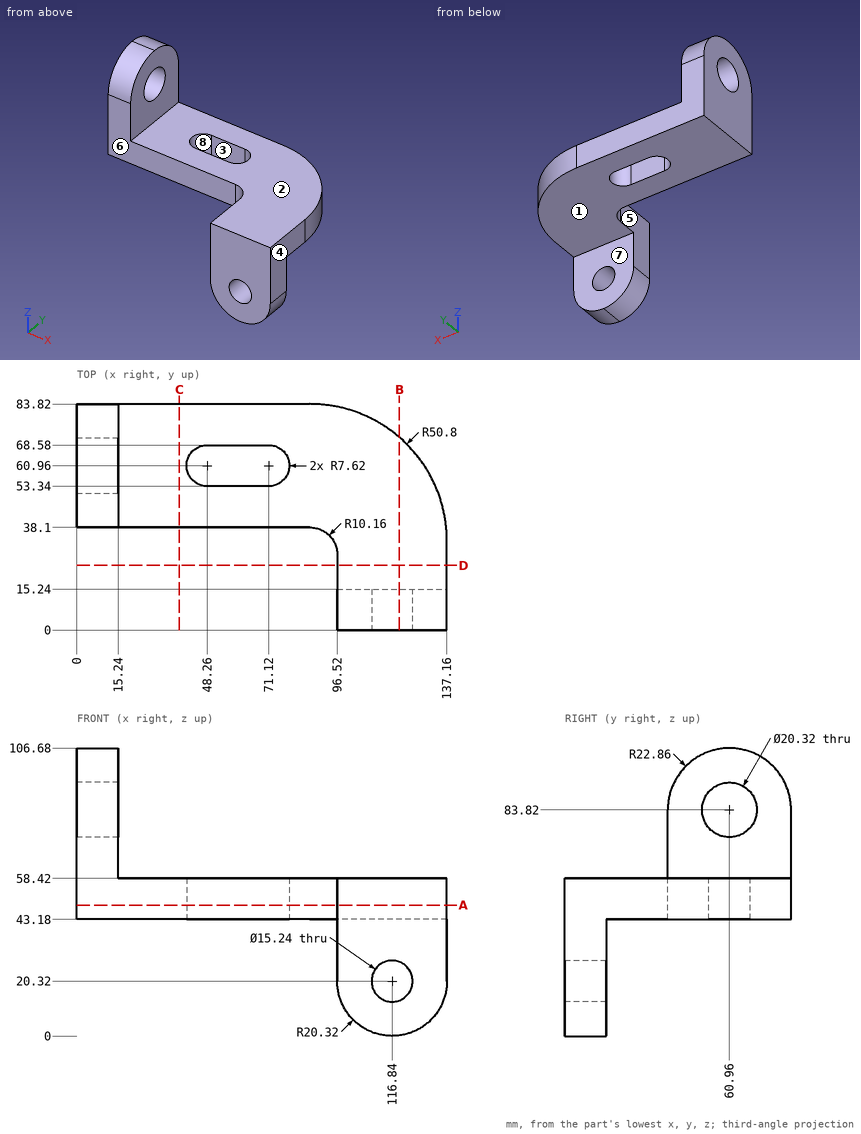
The figure shows three views and two pictorial views of one solid part (mm, origin at its lowest corner). Answer the questions. A direction names the side the tool comes from. Coordinates: 2 decimals unless noted, no trailing zeros. Order: outer loops, then holes, each group sorted by start corner. A loop starts at its lowest first (then second) coordinate and runs counter-clockwise, first axis right, second up.
Q1. A cutting plane is placed at D-D, the plane y = 24. Write down the section's boundary in (x, z), and give its area (3 significant figures).
Q2. Which of the six approach directions +Z, -Z, +X, -X, +Y, -Y give full straight-line access (tool end or side, diameter ignored) to the marked faces 1, 2, 3 and 4?
Q3. For a pull along Y with two mould halves and no side action, classify the marked faces 5, 6, 7 and 8 as pulls with the +Y half, pulls with the -Y half, needs draft (parallel to the pull), parting line crosses it, or undercut.
Q4. A cutting plane is placed at C-C, the plane x = 38. Write down the section's boundary in (y, z), and give its area (3 significant figures).
Q5. Consider line 1 (Z direction, x = 116.84, y = 9); line 2 (X direction, y = 12, z = 20); line 3 (X direction, y = 79.5, z = 91.5). Determine where each line is inside the solid, lowest interval first.
Q6. A cutting plane is placed at A-A, the plane z = 48.5. Write down the section's boundary in (x, y), and give its area (3 significant figures).
Q7. A cutting plane is placed at B-B, the plane x = 119.5. Write down the section's boundary in (y, z).
Q8. Given P1, Ø10, axis at x = 68, y = 73.5, coming from the -Z side; P2, Ø14, axis at y = 17, z = 43, coming from the -X side; P3, Ø12, axis at x = 43.5, z = 53.5, coming from the -Y side, each flat-ended and moving along its own axis, determine where each tip first touches the part or whether it passes through.
Answers follow:
1. outline: (96.52, 43.18) - (137.16, 43.18) - (137.16, 58.42) - (96.52, 58.42) - close
1. area: 619 mm2
2. face 1: -Z, +X, -X, +Y
2. face 2: +Z, +X, +Y, -Y
2. face 3: +Z, -Z
2. face 4: +Z, -Z, +X, +Y, -Y
3. face 5: needs draft
3. face 6: pulls with the -Y half
3. face 7: pulls with the +Y half
3. face 8: undercut
4. outline: (38.1, 43.18) - (83.82, 43.18) - (83.82, 58.42) - (38.1, 58.42) - close
4. area: 697 mm2
5. line 1: z = 0 to 12.7, 27.94 to 58.42
5. line 2: x = 96.52 to 109.23, 124.45 to 137.16
5. line 3: x = 0 to 15.24
6. outline: (0, 38.1) - (86.36, 38.1) arc R10.16 cw to (96.52, 27.94) - (96.52, 0) - (137.16, 0) - (137.16, 33.02) arc R50.8 ccw to (86.36, 83.82) - (0, 83.82) - close; hole (48.26, 53.34) - (71.12, 53.34) arc R7.62 ccw to (71.12, 68.58) - (48.26, 68.58) arc R7.62 ccw to start
6. area: 6,760 mm2
7. outline: (0, 0.17) - (15.24, 0.17) - (15.24, 13.18) - (0, 13.18) - close; (0, 27.46) - (15.24, 27.46) - (15.24, 43.18) - (71.52, 43.18) - (71.52, 58.42) - (0, 58.42) - close
8. P1: stops at z = 43.18
8. P2: stops at x = 96.52
8. P3: stops at y = 38.1
